```python
from build123d import *

# Parameters (mm, degrees)
CYLINDER006_R     = 1
CYLINDER006_DEPTH = 13
CYLINDER007_R     = 1
CYLINDER007_DEPTH = 13
CYLINDER008_R     = 1
CYLINDER008_DEPTH = 13
CYLINDER005_R     = 1
CYLINDER005_DEPTH = 13
CYLINDER009_R     = 1
CYLINDER009_DEPTH = 13
CYLINDER001_R     = 2
CYLINDER001_DEPTH = 13
CYLINDER002_R     = 2
CYLINDER002_DEPTH = 13
CYLINDER003_R     = 2
CYLINDER003_DEPTH = 13
CYLINDER004_R     = 2
CYLINDER004_DEPTH = 13
BOX001_W          = 10
BOX001_H          = 17
BOX001_DEPTH      = 8
BOX002_W          = 10
BOX002_H          = 17
BOX002_DEPTH      = 8
BOX003_W          = 10
BOX003_H          = 17
BOX003_DEPTH      = 8
BOX004_W          = 10
BOX004_H          = 17
BOX004_DEPTH      = 8
BOX005_W          = 10
BOX005_H          = 17
BOX005_DEPTH      = 8
BOX_W             = 100
BOX_H             = 44
BOX_DEPTH         = 16.5
BOX006_W          = 104
BOX006_H          = 48
BOX006_DEPTH      = 13
FILLET_R          = 4
CYLINDER_R        = 2
CYLINDER_DEPTH    = 13


with BuildPart() as cylinder006:
    # Cylinder006 → Cylinder006 (new body)
    with BuildSketch(Plane(origin=(20, -2, 0), x_dir=(1, 0, 0), z_dir=(0, 0, 1))):
        Circle(CYLINDER006_R)
    extrude(amount=CYLINDER006_DEPTH)


with BuildPart() as cylinder007:
    # Cylinder007 → Cylinder007 (new body)
    with BuildSketch(Plane(origin=(80, -2, 0), x_dir=(1, 0, 0), z_dir=(0, 0, 1))):
        Circle(CYLINDER007_R)
    extrude(amount=CYLINDER007_DEPTH)


with BuildPart() as cylinder008:
    # Cylinder008 → Cylinder008 (new body)
    with BuildSketch(Plane(origin=(48, 46, 0), x_dir=(1, 0, 0), z_dir=(0, 0, 1))):
        Circle(CYLINDER008_R)
    extrude(amount=CYLINDER008_DEPTH)


with BuildPart() as cylinder005:
    # Cylinder005 → Cylinder005 (new body)
    with BuildSketch(Plane(origin=(-2, 22, 0), x_dir=(1, 0, 0), z_dir=(0, 0, 1))):
        Circle(CYLINDER005_R)
    extrude(amount=CYLINDER005_DEPTH)


with BuildPart() as cylinder009:
    # Cylinder009 → Cylinder009 (new body)
    with BuildSketch(Plane(origin=(102, 22, 0), x_dir=(1, 0, 0), z_dir=(0, 0, 1))):
        Circle(CYLINDER009_R)
    extrude(amount=CYLINDER009_DEPTH)


with BuildPart() as cylinder001:
    # Cylinder001 → Cylinder001 (new body)
    with BuildSketch(Plane(origin=(80, -2, 0), x_dir=(1, 0, 0), z_dir=(0, 0, 1))):
        Circle(CYLINDER001_R)
    extrude(amount=CYLINDER001_DEPTH)


with BuildPart() as cylinder002:
    # Cylinder002 → Cylinder002 (new body)
    with BuildSketch(Plane(origin=(48, 46, 0), x_dir=(1, 0, 0), z_dir=(0, 0, 1))):
        Circle(CYLINDER002_R)
    extrude(amount=CYLINDER002_DEPTH)


with BuildPart() as cylinder003:
    # Cylinder003 → Cylinder003 (new body)
    with BuildSketch(Plane(origin=(-2, 22, 0), x_dir=(1, 0, 0), z_dir=(0, 0, 1))):
        Circle(CYLINDER003_R)
    extrude(amount=CYLINDER003_DEPTH)


with BuildPart() as cylinder004:
    # Cylinder004 → Cylinder004 (new body)
    with BuildSketch(Plane(origin=(102, 22, 0), x_dir=(1, 0, 0), z_dir=(0, 0, 1))):
        Circle(CYLINDER004_R)
    extrude(amount=CYLINDER004_DEPTH)


with BuildPart() as box001:
    # Box001 → Box001 (new body)
    with BuildSketch(Plane(origin=(1.6, 37, 0), x_dir=(1, 0, 0), z_dir=(0, 0, 1))):
        with Locations((5, 8.5)):
            Rectangle(BOX001_W, BOX001_H)
    extrude(amount=BOX001_DEPTH)


with BuildPart() as box002:
    # Box002 → Box002 (new body)
    with BuildSketch(Plane(origin=(13.8, 37, 0), x_dir=(1, 0, 0), z_dir=(0, 0, 1))):
        with Locations((5, 8.5)):
            Rectangle(BOX002_W, BOX002_H)
    extrude(amount=BOX002_DEPTH)


with BuildPart() as box003:
    # Box003 → Box003 (new body)
    with BuildSketch(Plane(origin=(25.8, 37, 0), x_dir=(1, 0, 0), z_dir=(0, 0, 1))):
        with Locations((5, 8.5)):
            Rectangle(BOX003_W, BOX003_H)
    extrude(amount=BOX003_DEPTH)


with BuildPart() as box004:
    # Box004 → Box004 (new body)
    with BuildSketch(Plane(origin=(58.8, 37, 0), x_dir=(1, 0, 0), z_dir=(0, 0, 1))):
        with Locations((5, 8.5)):
            Rectangle(BOX004_W, BOX004_H)
    extrude(amount=BOX004_DEPTH)


with BuildPart() as box005:
    # Box005 → Box005 (new body)
    with BuildSketch(Plane(origin=(93.8, 42, 0), x_dir=(0, -1, 0), z_dir=(0, 0, 1))):
        with Locations((5, 8.5)):
            Rectangle(BOX005_W, BOX005_H)
    extrude(amount=BOX005_DEPTH)


with BuildPart() as fusion:
    # Box → Box (new body)
    with BuildSketch(Plane.XY.offset(-5)):
        with Locations((50, 22)):
            Rectangle(BOX_W, BOX_H)
    extrude(amount=BOX_DEPTH)

    # Fusion: union Box001, Box002, Box003, Box004, Box005
    add(box001.part)
    add(box002.part)
    add(box003.part)
    add(box004.part)
    add(box005.part)


with BuildPart() as fillet_body:
    # Box006 → Box006 (new body)
    with BuildSketch(Plane(origin=(-2, -2, 0), x_dir=(1, 0, 0), z_dir=(0, 0, 1))):
        with Locations((52, 24)):
            Rectangle(BOX006_W, BOX006_H)
    extrude(amount=BOX006_DEPTH)

    # Cut: cut Fusion
    add(fusion.part, mode=Mode.SUBTRACT)

    # Fillet
    fillet_edges = [fillet_body.edges().sort_by_distance(p)[0] for p in [
        (-2, -2, 6.5),
        (-2, 46, 6.5),
        (102, -2, 6.5),
        (102, 46, 6.5),
    ]]
    fillet(fillet_edges, radius=FILLET_R)


with BuildPart() as cut006:
    # Cylinder → Cylinder (new body)
    with BuildSketch(Plane(origin=(20, -2, 0), x_dir=(1, 0, 0), z_dir=(0, 0, 1))):
        Circle(CYLINDER_R)
    extrude(amount=CYLINDER_DEPTH)

    # Fusion002: union Cylinder001, Cylinder002, Cylinder003, Cylinder004, Fillet body
    add(cylinder001.part)
    add(cylinder002.part)
    add(cylinder003.part)
    add(cylinder004.part)
    add(fillet_body.part)

    # Cut002: cut Cylinder009
    add(cylinder009.part, mode=Mode.SUBTRACT)

    # Cut003: cut Cylinder005
    add(cylinder005.part, mode=Mode.SUBTRACT)

    # Cut004: cut Cylinder008
    add(cylinder008.part, mode=Mode.SUBTRACT)

    # Cut005: cut Cylinder007
    add(cylinder007.part, mode=Mode.SUBTRACT)

    # Cut006: cut Cylinder006
    add(cylinder006.part, mode=Mode.SUBTRACT)


solid = cut006.part
```
Verification items for the finished model (mm, model axes). A direction names the side the tool comes from. Give positions to 0.01 mm unless a question says otherwise; leave off trailing zeros. Order: outer loops, then holes, each group sorted by start corner. A loop starts at its lowest first (then second) coordinate and runs counter-clockwise, first axis right, second up. Notation, with made-up numbers: (40.5, 70) - (69.5, 70) arc R16 ccw to (69.5, 100) - close; hole circle Ø5 at (34.25, 44). An arc over 180 degrees is marked (long way). Answer as CSV lines item,"result". Start each with the question number.
Item 1: Access from +Z, -Z, +X, -X, +Y, -Y to the whole of each face (thin tool, end or side, straight path). Record for faces 1 (the face through (102, 11, 6)), 2 (the face through (49, 0, 6)), 3 (the face through (68.8, 45, 4)), 4 (the face through (101, 37, 8)).
Item 2: Section check B-B, the plane z = 10.5. Record the boundary of the cut face in (x, y).
Item 3: Section check D-D, the plane y = 40. Record the boundary of the cut face in (x, z).
Item 4: Material ranges on L1, parallel to Y at x = 20, z = 10.25; L2, parallel to Y at x = 48, z = 3.5; L3, parallel to Y at x = 91, z = 5.75, recorded low to high.
Item 5: Section check A-A, the plane x = 80. Record the boundary of the cut face in (y, z), plus the area to 3 significant figures.
Item 6: Gauge pin test, flat ends, axial feed: pin 1 (3 mm diameter, centred on y = 9, z = 10.5, fed in from +X); pin 2 (1 mm diameter, centred on x = 28.5, y = 44.5, fed in from -Z); pin 3 (1.5 mm diameter, centred on x = 40, z = 7, fed in from +Y); pin 4 (4 mm diameter, centred on x = 18, z = 10, fed in from -Y). Record the tip position at first contact, or that the pin passes through.
Item 7: Mould release check, pull along Y, two halves, no side actions. Record for faces 5 (the face through (64, 45, 8)), 6 (the face through (100.797, -0.859, 6.591)), 7 (the face through (-2, 21, 6)): released by +Y, released by -Y, zero draft, split by the parting line, or undercut.
Item 8: Section check C-C, the plane y = 22. Record the boundary of the cut face in (x, z), plus the area to 3 significant figures.
Filled in:
1,face 1,"+Z, -Z, +X, -Y"
1,face 2,"-Z"
1,face 3,"-Z, +Y"
1,face 4,"-Z, +X"
2,outline,"(-2, 2) arc R4 ccw to (2, -2) - (18, -2) arc R2 ccw to (22, -2) - (78, -2) arc R2 ccw to (82, -2) - (98, -2) arc R4 ccw to (102, 2) - (102, 20) arc R2 ccw to (102, 24) - (102, 42) arc R4 ccw to (98, 46) - (50, 46) arc R2 ccw to (46, 46) - (2, 46) arc R4 ccw to (-2, 42) - (-2, 24) arc R2 ccw to (-2, 20) - close; hole circle Ø2 at (-2, 22); hole (0, 0) - (100, 0) - (100, 44) - (0, 44) - close; hole circle Ø2 at (20, -2); hole circle Ø2 at (48, 46); hole circle Ø2 at (80, -2); hole circle Ø2 at (102, 22)"
3,outline,"(-2, 0) - (0, 0) - (0, 11.5) - (100, 11.5) - (100, 8) - (102, 8) - (102, 13) - (-2, 13) - close"
4,L1,"-4 to -3, -1 to 0, 44 to 46"
4,L2,"-2 to 0, 44 to 45, 47 to 48"
4,L3,"-2 to 0, 44 to 46"
5,outline,"(-4, 0) - (-3, 0) - (-3, 13) - (-4, 13) - close; (-1, 0) - (0, 0) - (0, 11.5) - (44, 11.5) - (44, 0) - (46, 0) - (46, 13) - (-1, 13) - close"
5,area,"118 mm^2"
6,pin 1,"x = 102"
6,pin 2,"z = 8"
6,pin 3,"y = 46"
6,pin 4,"y = -4"
7,face 5,"zero draft"
7,face 6,"released by -Y"
7,face 7,"undercut"
8,outline,"(-4, 0) - (-3, 0) - (-3, 13) - (-4, 13) - close; (-1, 0) - (0, 0) - (0, 11.5) - (100, 11.5) - (100, 0) - (101, 0) - (101, 13) - (-1, 13) - close; (103, 0) - (104, 0) - (104, 13) - (103, 13) - close"
8,area,"202 mm^2"
